```python
from build123d import *

# Parameters (mm, degrees)
F0_W           = 78.74
F0_H           = 17.78
F1_DEPTH       = 4.445
F2_W           = 19.05
F2_H           = 78.74
F3_DEPTH       = 4.445
F4_R           = 8.88999
F6_D           = 4.4958
F6_CSINK_D     = 9.1186
F6_CSINK_ANGLE = 82
F7_R           = 8.89
F8_DEPTH       = 4.446


# Not quite as in the source:
# - a fillet or chamfer is up to 0.001 mm smaller than in the source, because OpenCascade refuses the exact size


with BuildPart() as f1:
    # F0 (on Top) → F1 (new body)
    with BuildSketch(Plane.XY):
        Rectangle(F0_W, F0_H)
    extrude(amount=F1_DEPTH)

    # F2 (on Top) → F3 (join, through all)
    with BuildSketch(Plane.XY):
        Rectangle(F2_W, F2_H)
    extrude(amount=F3_DEPTH)

    # F4 (radius 8.89 in the source; OpenCascade refuses exactly that, so slightly less here)
    f4_edges = [f1.edges().sort_by_distance(p)[0] for p in [
        (9.525, -39.37, 2.2225),
        (-9.525, -39.37, 2.2225),
        (39.37, -8.89, 2.2225),
        (39.37, 8.89, 2.2225),
        (9.525, 39.37, 2.2225),
        (-39.37, -8.89, 2.2225),
        (-39.37, 8.89, 2.2225),
        (-9.525, 8.89, 2.2225),
        (-9.525, 39.37, 2.2225),
        (-9.525, -8.89, 2.2225),
        (9.525, -8.89, 2.2225),
        (9.525, 8.89, 2.2225),
    ]]
    fillet(f4_edges, radius=F4_R)

    # F6 (through all)
    with Locations(Plane.XY.offset(4.445)):
        with Locations((34.29, 0), (0, -34.29), (-34.29, 0), (0, 34.29)):
            CounterSinkHole(F6_D / 2, F6_CSINK_D / 2, counter_sink_angle=F6_CSINK_ANGLE)

    # F7 (on Top) → F8 (cut, through all)
    with BuildSketch(Plane.XY):
        Circle(F7_R)
    extrude(amount=F8_DEPTH, mode=Mode.SUBTRACT)


solid = f1.part
```
Input: part model. Units: mm. Frame: model coordinates. A direction names the side the tool comes from. Coordinates: 2 decimals unless noted, no trailing zeros. Loops run counter-clockwise (first coordinate to the right, second up) from the corner with the lowest first, then second, coordinate; pieces in that order, holes last. Notation, with made-up numbers: (19.25, -7) -> (52.25, -7) arc R21 cw to (52.25, 17) -> close; hole circle Ø5 at (88.5, 87.5). An arc over 180 degrees is marked (long way). Use a Markdown table: item, result.
1) Access query for faces 1 (the flat face through (24, -8.89, 2)), 2 (the flat face through (24, 8.89, 2)), 3 (the flat face through (-25, -8.89, 2)), 4 (the flat face through (-25, 8.89, 2)), 5 (the cylindrical face through (0.487, -36.484, 0.881)). Directions: +Z, -Z, +X, -X, +Y, -Y. A direction counts if a zero-diameter tool reaches every point of the face in a straight line with its end or side. Return the directions, or none.
Results found:
| item | result |
|---|---|
| face 1 | +Z, -Z, +X, -Y |
| face 2 | +Z, -Z, +X, +Y |
| face 3 | +Z, -Z, -X, -Y |
| face 4 | +Z, -Z, -X, +Y |
| face 5 | +Z, -Z |
2) Material intervals for line 1 along X through (y, z) = (0, 0.7); line 2 along X through (y, z) = (-1, 3.45), sorted ascending. Write a range as from..to.
Results found:
| item | result |
|---|---|
| line 1 | x = -39.37..-36.54, -32.04..-8.89, 8.89..32.04, 36.54..39.37 |
| line 2 | x = -39.31..-37.85, -30.73..-8.83, 8.83..30.73, 37.85..39.31 |
3) Cut plane D-D (x = -34.29). Return the cut outline in (y, z) (3 decimals), then the cut area to 3 significant figures.
Results found:
| item | result |
|---|---|
| outline | (-8.032, 0) -> (-2.248, 0) -> (-2.248, 1.786) -> (-4.559, 4.445) -> (-8.032, 4.445) -> close; (2.248, 0) -> (8.032, 0) -> (8.032, 4.445) -> (4.559, 4.445) -> (2.248, 1.786) -> close |
| area | 45.3 mm2 |
4) Cut plane C-C (x = -6). Return the cut outline in (y, z) (3 decimals), then the cut area to 3 significant figures.
Results found:
| item | result |
|---|---|
| outline | (-37.569, 0) -> (-6.56, 0) -> (-6.56, 4.445) -> (-37.569, 4.445) -> close; (6.56, 0) -> (37.569, 0) -> (37.569, 4.445) -> (6.56, 4.445) -> close |
| area | 276 mm2 |
5) Contact query for flat-ended pins moving along their axis: pin 1 (3.5 mm diameter, centred on x = 0, y = -34.29, fed in from +Z); pin 2 (6 mm diameter, centred on x = 0, y = 34.29, fed in from +Z); pin 3 (6 mm diameter, centred on x = 12.5, y = 17, fed in from -Z); pin 4 (2 mm diameter, centred on x = 23.5, z = 1.5, fed in from -Y). Output: stop coordinate, or through.
Results found:
| item | result |
|---|---|
| pin 1 | passes through |
| pin 2 | stops at z = 2.65 |
| pin 3 | stops at z = 0 |
| pin 4 | stops at y = -8.89 |
6) Pull-direction query (Y, two-part tool) for faces 6 (the flat face through (3, 9, 0)), 7 (the conical face through (-36.47, -0.904, 1.915)), 8 (the conical face through (0.512, 31.986, 1.915)), 9 (the cylindrical face through (-36.83, 6.22, 2.25)); classes: released by +Y, released by -Y, zero draft, split by the parting line, or undercut.
Results found:
| item | result |
|---|---|
| face 6 | zero draft |
| face 7 | undercut |
| face 8 | undercut |
| face 9 | released by +Y |
7) Cut plane A-A (z = 0.95). Give the number of separate pieces and of enclosed holes in the cut face, then the cut area to 3 significant figures.
Results found:
| item | result |
|---|---|
| separate pieces | 1 |
| enclosed holes | 5 |
| area | 2,180 mm2 |
8) Cut plane B-B (y = -34.29). Return the cut outline in (x, z) (3 decimals), then the cut area to 3 significant figures.
Results found:
| item | result |
|---|---|
| outline | (-8.667, 0) -> (-2.248, 0) -> (-2.248, 1.786) -> (-4.559, 4.445) -> (-8.667, 4.445) -> close; (2.248, 0) -> (8.667, 0) -> (8.667, 4.445) -> (4.559, 4.445) -> (2.248, 1.786) -> close |
| area | 50.9 mm2 |
